Answer from the drawing. Dimensions are ordinates in mm from the lowest x, y and z of the part. A direction names the side the tool comes from. Give positions to 0.01 mm unless a question says otherwise; leave off trailing zeros. Write each loop counter-clockwise with the first axis right and the second up, starting at its lowest first coordinate (ties: lowest second). Pieces come first, ordered by that corner, then holes.
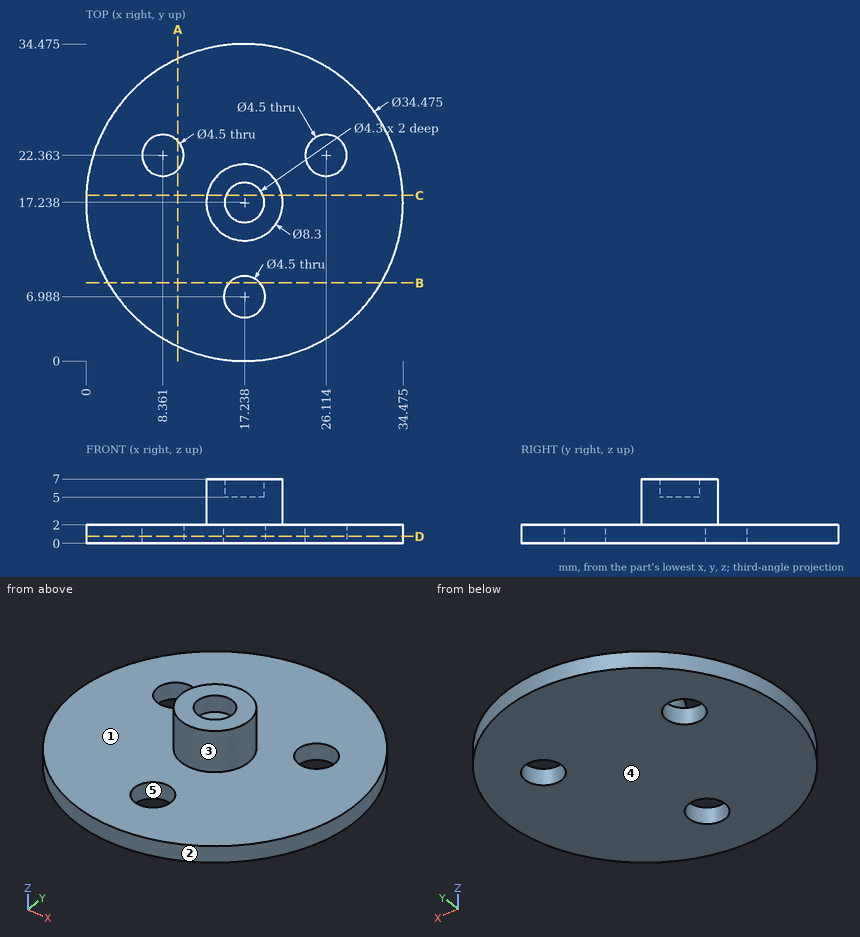
Item 1: Section C-C (y = 18) is taken. Write down the section's boundary in (x, z), and give its area (3 significant figures).
Result set:
outline: (0.02, 0) - (34.46, 0) - (34.46, 2) - (21.32, 2) - (21.32, 7) - (19.25, 7) - (19.25, 5) - (15.23, 5) - (15.23, 7) - (13.16, 7) - (13.16, 2) - (0.02, 2) - close
area: 102 mm2
Item 2: Section D-D (z = 0.75) is taken. Give the number of separate pieces and of enclosed holes in the cut face, and give its area (3 significant figures).
Result set:
separate pieces: 1
enclosed holes: 3
area: 886 mm2
Item 3: Determine the mould class of the marked faces 3, 4 and 5 for opening direction X: pulls with the +X half, pulls with the -X half, needs draft (parallel to the pull), parting line crosses it, or undercut.
Result set:
face 3: parting line crosses it
face 4: needs draft
face 5: undercut
Item 4: Section A-A (x = 10) is taken. Write down the section's boundary in (y, z).
Result set:
outline: (1.59, 0) - (20.82, 0) - (20.82, 2) - (1.59, 2) - close; (23.9, 0) - (32.88, 0) - (32.88, 2) - (23.9, 2) - close
Item 5: Which of the six approach directions +Z, -Z, +X, -X, +Y, -Y give full straight-line access (tool end or side, diameter ignored) to the marked faces 1 and 2?
Result set:
face 1: +Z
face 2: +Z, -Z
Item 6: Find the intervals of material crossed by line 1 along Z through (x, y) = (24, 3); line 2 along X through (y, z) = (17, 2.25) (1 decimal); line 3 along Y through (x, z) = (9, 1.25) (1 decimal), in increasing order.
Result set:
line 1: z = 0 to 2
line 2: x = 13.1 to 21.4
line 3: y = 2.1 to 20.2, 24.5 to 32.4
Item 7: Each of these flat-tipped pins is pushed along its axis until it touches: pin 1 Ø1.5 at (x, y) = (11, 8) entering from -Z; pin 2 Ø1.5 at (x, z) = (26.5, 1.5) entering from +Y; pin 3 Ø3.5 at (x, y) = (8.36, 22.36) entering from -Z; pin 4 Ø2 at (x, y) = (17, 16.5) entering from +Z. Where does it stop, or does it pass through?
Result set:
pin 1: stops at z = 0
pin 2: stops at y = 32.23
pin 3: passes through
pin 4: stops at z = 5
Item 8: Section B-B (y = 8.5) is taken. Write down the section's boundary in (x, z).
Result set:
outline: (2.38, 0) - (15.57, 0) - (15.57, 2) - (2.38, 2) - close; (18.9, 0) - (32.1, 0) - (32.1, 2) - (18.9, 2) - close
